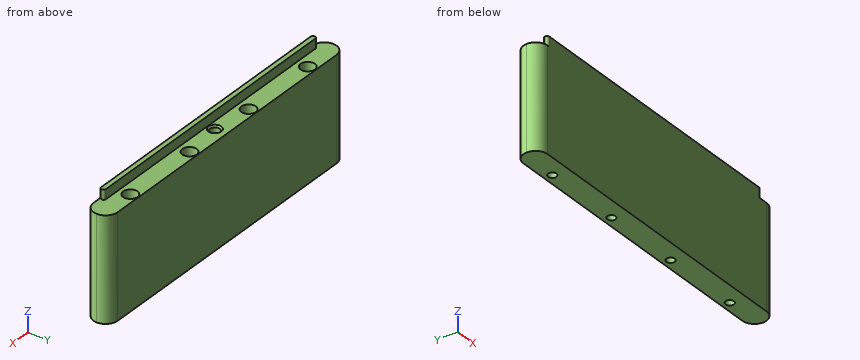
```python
from build123d import *

# Parameters (mm, degrees)
SKETCH1_W           = 200
SKETCH1_H           = 15
SKETCH1_R           = 2.6
BOSS_EXTRUDE1_DEPTH = 64
SKETCH2_R           = 4.5
CUT_EXTRUDE1_DEPTH  = 57
FILLET3_R           = 7.5
SKETCH3_W           = 180
SKETCH3_H           = 3
BOSS_EXTRUDE2_DEPTH = 6
FILLET4_R           = 1.5
SKETCH4_R           = 3.05
CUT_EXTRUDE2_DEPTH  = 8
CHAMFER1_SIZE       = 1


with BuildPart() as part:
    # Sketch1 → Boss-Extrude1 (new body)
    with BuildSketch(Plane.XY):
        Rectangle(SKETCH1_W, SKETCH1_H)
        with Locations((75, 2.5)):
            Circle(SKETCH1_R, mode=Mode.SUBTRACT)
        with Locations((25, 2.5)):
            Circle(SKETCH1_R, mode=Mode.SUBTRACT)
        with Locations((-25, 2.5)):
            Circle(SKETCH1_R, mode=Mode.SUBTRACT)
        with Locations((-75, 2.5)):
            Circle(SKETCH1_R, mode=Mode.SUBTRACT)
    extrude(amount=BOSS_EXTRUDE1_DEPTH)

    # Sketch2 → Cut-Extrude1 (cut)
    with BuildSketch(Plane.XY.offset(64)):
        with Locations((-75, 2.5)):
            Circle(SKETCH2_R)
        with Locations((-25, 2.5)):
            Circle(SKETCH2_R)
        with Locations((25, 2.5)):
            Circle(SKETCH2_R)
        with Locations((75, 2.5)):
            Circle(SKETCH2_R)
    extrude(amount=-CUT_EXTRUDE1_DEPTH, mode=Mode.SUBTRACT)

    # Fillet3
    fillet3_edges = [part.edges().sort_by_distance(p)[0] for p in [
        (100, 7.5, 32),
        (100, -7.5, 32),
        (-100, 7.5, 32),
        (-100, -7.5, 32),
    ]]
    fillet(fillet3_edges, radius=FILLET3_R - 0.0001)  # a hair under: the kernel refuses the full size

    # Sketch3 → Boss-Extrude2 (add)
    with BuildSketch(Plane.XY.offset(64)):
        with Locations((-2.5, -6)):
            Rectangle(SKETCH3_W, SKETCH3_H)
    extrude(amount=BOSS_EXTRUDE2_DEPTH)

    # Fillet4
    fillet4_edges = [part.edges().sort_by_distance(p)[0] for p in [
        (87.5, -4.5, 67),
        (87.5, -7.5, 67),
        (-92.5, -7.5, 67),
        (-92.5, -4.5, 67),
    ]]
    fillet(fillet4_edges, radius=FILLET4_R - 0.0001)  # a hair under: the kernel refuses the full size

    # Sketch4 → Cut-Extrude2 (cut)
    with BuildSketch(Plane.XY.offset(64)):
        with Locations((0.125314072, 0)):
            Circle(SKETCH4_R)
    extrude(amount=-CUT_EXTRUDE2_DEPTH, mode=Mode.SUBTRACT)

    # Chamfer1
    chamfer1_edges = [part.edges().sort_by_distance(p)[0] for p in [
        (-2.924685928, 0, 64),
    ]]
    chamfer(chamfer1_edges, length=CHAMFER1_SIZE)


solid = part.part
```
Here's how the part is built. I have some questions about the finished solid (model axes, mm). Coordinates: 2 decimals unless noted, no trailing zeros. Order: outer loops, then holes, each group sorted by start corner. A loop starts at its lowest first (then second) coordinate and runs counter-clockwise, first axis right, second up.
1) Imagine slicing it at C-C on x = 7.5. List the corners of the cut face in (y, z) for me, and give its area (3 significant figures).
2) I need wall thicknesses on line 1 (X direction, y = -1.5, z = 15); line 2 (X direction, y = 2.5, z = 3.25); line 3 (Y direction, x = -75, z = 29). Which ranges of each line are inside material? Lowest first, please.
3) Will these pins go through, and if not, where does the flat tip stop? pin 1 (7 mm diameter, centred on x = 26.5, y = 1.5, fed in from +Z); pin 2 (2.5 mm diameter, centred on x = 73.5, y = 1, fed in from +Z); pin 3 (5 mm diameter, centred on y = 3.5, z = 55.5, fed in from +X).
4) Imagine slicing it at B-B on z = 20.5. State how many separate pieces and enclosed holes the cut face has, and give its area (3 significant figures).
5) Imagine slicing it at A-A on x = -25. List the corners of the cut face in (y, z) for me, and give its area (3 significant figures).
Response values:
1. outline: (-7.5, 0) - (7.5, 0) - (7.5, 64) - (-4.5, 64) - (-4.5, 70) - (-7.5, 70) - close
1. area: 978 mm2
2. line 1: x = -99.85 to -77.06, -72.94 to -27.06, -22.94 to 22.94, 27.06 to 72.94, 77.06 to 99.85
2. line 2: x = -99.57 to -77.6, -72.4 to -27.6, -22.4 to 22.4, 27.6 to 72.4, 77.6 to 99.57
2. line 3: y = -7.5 to -2, 7 to 7.5
3. pin 1: stops at z = 64
3. pin 2: stops at z = 7
3. pin 3: stops at x = 99.93
4. separate pieces: 1
4. enclosed holes: 4
4. area: 2,700 mm2
5. outline: (-7.5, 0) - (-0.1, 0) - (-0.1, 7) - (-2, 7) - (-2, 64) - (-4.5, 64) - (-4.5, 70) - (-7.5, 70) - close; (5.1, 0) - (7.5, 0) - (7.5, 64) - (7, 64) - (7, 7) - (5.1, 7) - close
5. area: 429 mm2
